```python
from build123d import *

# Parameters (mm, degrees)
SKETCH_1_W                  = 20
SKETCH_1_H                  = 20
EXTRUDE_1_DEPTH             = 15
SKETCH_2_W                  = 17
SKETCH_2_H                  = 12
CUT_EXTRUDE_1_DEPTH         = 49.176757882
HOLE_WIZARD_4_2_4_2_1_D     = 4.2
HOLE_WIZARD_4_2_4_2_1_DEPTH = 15
HOLE_WIZARD_4_0_4_1_D       = 4


with BuildPart() as part:
    # 草图1 → 凸台-拉伸1 (new body)
    with BuildSketch(Plane.XZ.offset(25)):
        with Locations((-26, 10)):
            Rectangle(SKETCH_1_W, SKETCH_1_H)
    extrude(amount=-EXTRUDE_1_DEPTH)

    # 草图2 → 切除-拉伸1 (cut, through all)
    with BuildSketch(Plane(origin=(0, 0, 0), x_dir=(-1, 0, 0), z_dir=(0, 0, -1))):
        with Locations((24.5, -19)):
            Rectangle(SKETCH_2_W, SKETCH_2_H)
    extrude(amount=-CUT_EXTRUDE_1_DEPTH, mode=Mode.SUBTRACT)

    # Ø4.2 (4.2) 直径孔1
    with Locations(Plane(origin=(0, -10, 0), x_dir=(1, 0, 0), z_dir=(0, 1, 0))):
        with Locations((-26, -10)):
            Hole(HOLE_WIZARD_4_2_4_2_1_D / 2, depth=HOLE_WIZARD_4_2_4_2_1_DEPTH)

    # Ø4.0 (4) 直径孔1 (through all)
    with Locations(Plane(origin=(-33, 0, 0), x_dir=(0, 0, -1), z_dir=(1, 0, 0))):
        with Locations((-15, -20), (-5, -20)):
            Hole(HOLE_WIZARD_4_0_4_1_D / 2)


solid = part.part
```
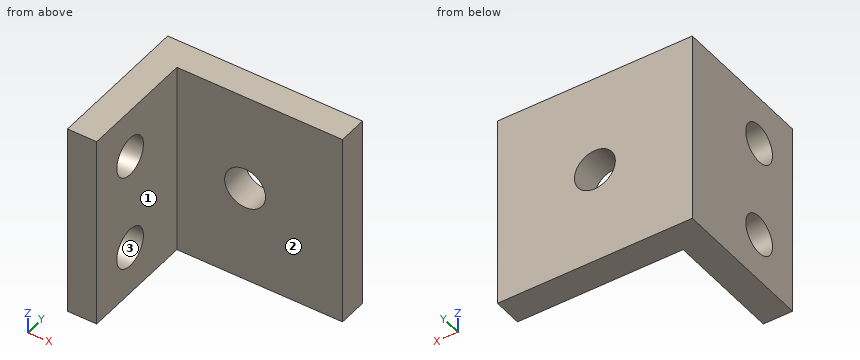
Part model, mm, in its own coordinate system. Face numbers are marked on the shaded views. Round coordinates to 2 decimals unless told otherwise and drop trailing zeros. Loops run counter-clockwise (first coordinate to the right, second up) from the corner with the lowest first, then second, coordinate; pieces in that order, holes last. Notation, with made-up numbers: (-23.75, 66) -> (-1.75, 66) arc R23 cw to (-1.75, 90) -> close; hole circle Ø9 at (74.5, 6). An arc over 180 degrees is marked (long way). Use CSV: the item, a comma, the result in double quotes. Start each with the question number.
1) Cut at A-A, the plane z = 10. Write the cut outline in (x, y).
2) Pull direction Y, two halves, no side cores. Call the marked faces 1, 2 and 3: +Y half, -Y half, draft (parallel to the pull), parting line (faces both ways), or undercut.
3) Cut at C-C, the plane y = -12.5. Write the cut outline in (x, z).
4) Wall check: L1, parallel to Y at x = -35.1, z = 15; L2, parallel to X at y = -11.7, z = 10; L3, parallel to Y at x = -20.5, z = 8.25. Give the ranges that are in metal, low to high. Write a range as [from, to].
5) Cut at B-B, the plane x = -26. Write the cut outline in (y, z).
6) Drop flat-ended pins along their axis: P1, Ø8, axis at x = -21.5, z = 14, coming from the -Y side; P2, Ø2, axis at y = -15, z = 12.5, coming from the +X side. Give the stop position or say it passes through.
7) Cut at D-D, the plane y = -20. Write the cut outline in (x, z).
Determined:
1,outline,"(-36, -25) -> (-33, -25) -> (-33, -13) -> (-28.1, -13) -> (-28.1, -10) -> (-36, -10) -> close; (-23.9, -13) -> (-16, -13) -> (-16, -10) -> (-23.9, -10) -> close"
2,face 1,"draft"
2,face 2,"-Y half"
2,face 3,"undercut"
3,outline,"(-36, 0) -> (-16, 0) -> (-16, 20) -> (-36, 20) -> close; hole circle Ø4.2 at (-26, 10)"
4,L1,"y = [-25, -22], [-18, -10]"
4,L2,"x = [-36, -28.1], [-23.9, -16]"
4,L3,"y = [-13, -10]"
5,outline,"(-13, 0) -> (-10, 0) -> (-10, 7.9) -> (-13, 7.9) -> close; (-13, 12.1) -> (-10, 12.1) -> (-10, 20) -> (-13, 20) -> close"
6,P1,"stops at y = -13"
6,P2,"stops at x = -33"
7,outline,"(-36, 0) -> (-33, 0) -> (-33, 3) -> (-36, 3) -> close; (-36, 7) -> (-33, 7) -> (-33, 13) -> (-36, 13) -> close; (-36, 17) -> (-33, 17) -> (-33, 20) -> (-36, 20) -> close"
